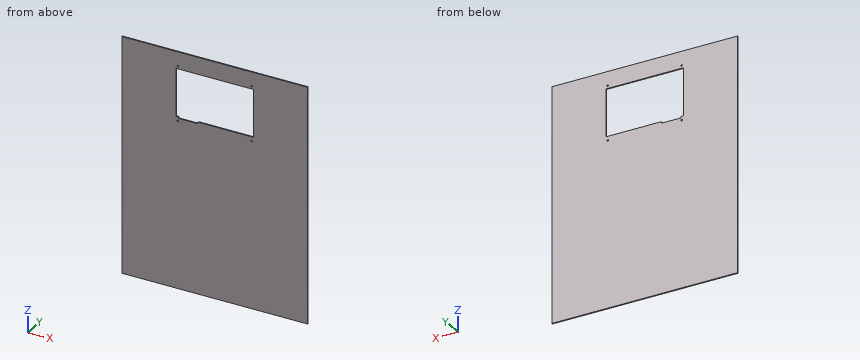
```python
from build123d import *

# Parameters (mm, degrees)
SKETCH1_W           = 395
SKETCH1_H           = 496
BOSS_EXTRUDE1_DEPTH = 2.5
CUT_EXTRUDE1_DEPTH  = 2.5
SKETCH6_R           = 1.65
CUT_EXTRUDE2_DEPTH  = 2.5


with BuildPart() as part:
    # Sketch1 → Boss-Extrude1 (new body)
    with BuildSketch(Plane(origin=(0, 0, 0), x_dir=(1, 0, 0), z_dir=(0, 1, 0))):
        Rectangle(SKETCH1_W, SKETCH1_H)
    extrude(amount=BOSS_EXTRUDE1_DEPTH)

    # Sketch4 → Cut-Extrude1 (cut)
    with BuildSketch(Plane(origin=(0, 2.5, 0), x_dir=(1, 0, 0), z_dir=(0, 1, 0))):
        with BuildLine():
            Line((-78.7, -112.1), (-82.2, -112.1))
            ThreePointArc((-82.2, -112.1), (-82.553553391, -112.246446609), (-82.7, -112.6))
            Line((-82.7, -112.6), (-82.7, -212))
            ThreePointArc((-82.7, -212), (-82.553553391, -212.353553391), (-82.2, -212.5))
            Line((-82.2, -212.5), (82.2, -212.5))
            ThreePointArc((82.2, -212.5), (82.553553391, -212.353553391), (82.7, -212))
            Line((82.7, -212), (82.7, -112.6))
            ThreePointArc((82.7, -112.6), (82.553553391, -112.246446609), (82.2, -112.1))
            Line((82.2, -112.1), (-34.7, -112.1))
            ThreePointArc((-34.7, -112.1), (-35.407106781, -111.807106781), (-35.7, -111.1))
            Line((-35.7, -111.1), (-35.7, -109.8))
            ThreePointArc((-35.7, -109.8), (-35.992893219, -109.092893219), (-36.7, -108.8))
            Line((-36.7, -108.8), (-76.7, -108.8))
            ThreePointArc((-76.7, -108.8), (-77.407106781, -109.092893219), (-77.7, -109.8))
            Line((-77.7, -109.8), (-77.7, -111.1))
            ThreePointArc((-77.7, -111.1), (-77.992893219, -111.807106781), (-78.7, -112.1))
        make_face()
    extrude(amount=-CUT_EXTRUDE1_DEPTH, mode=Mode.SUBTRACT)

    # Sketch6 → Cut-Extrude2 (cut)
    with BuildSketch(Plane(origin=(0, 2.5, 0), x_dir=(1, 0, 0), z_dir=(0, 1, 0))):
        with Locations((78.5, -103.4)):
            Circle(SKETCH6_R)
        with Locations((-78.5, -103.4)):
            Circle(SKETCH6_R)
        with Locations((-78.5, -218.3)):
            Circle(SKETCH6_R)
        with Locations((78.5, -218.3)):
            Circle(SKETCH6_R)
    extrude(amount=-CUT_EXTRUDE2_DEPTH, mode=Mode.SUBTRACT)


solid = part.part
```
Model file for the job. Use its own axes, mm. Coordinates: 2 decimals unless noted, no trailing zeros. Write each loop counter-clockwise with the first axis right and the second up, starting at its lowest first coordinate (ties: lowest second). Pieces come first, ordered by that corner, then holes. Notation, with made-up numbers: (51, -14) - (71, -14) arc R17 ccw to (71, -7) - close; hole circle Ø4 at (-2.5, -10.75). An arc over 180 degrees is marked (long way). One line per question, with ' | ' between items. Start each with the question number.
Q1. Cut at B-B, the plane x = -45.5. List the corners of the cut face in (y, z).
Q2. Pin check, flat tips, straight feed: pin 1 (2.5 mm diameter, centred on x = -78.5, z = 218.3, fed in from -Y); pin 2 (5.5 mm diameter, centred on x = 78.5, z = 218.3, fed in from +Y). Stop position of each tip, or through.
Q3. Drill centre lines: line 1 (Z direction, x = -78.5, y = 0.6); line 2 (X direction, y = 0.6, z = 103.4); line 3 (Z direction, x = 36, y = 1.6). Where is each one in solid material? Low to high. Write a range as [from, to].
Q4. Cut at A-A, the plane y = 1.05. List the corners of the cut face in (x, z).
Answer below:
1) outline: (0, -248) - (2.5, -248) - (2.5, 108.8) - (0, 108.8) - close; (0, 212.5) - (2.5, 212.5) - (2.5, 248) - (0, 248) - close
2) pin 1: through | pin 2: y = 2.5
3) line 1: [-248, 101.75], [105.05, 112.08], [212.5, 216.65], [219.95, 248] | line 2: [-197.5, -80.15], [-76.85, 76.85], [80.15, 197.5] | line 3: [-248, 112.1], [212.5, 248]
4) outline: (-197.5, -248) - (197.5, -248) - (197.5, 248) - (-197.5, 248) - close; hole (-82.7, 112.6) arc R0.5 ccw to (-82.2, 112.1) - (-78.7, 112.1) arc R1 cw to (-77.7, 111.1) - (-77.7, 109.8) arc R1 ccw to (-76.7, 108.8) - (-36.7, 108.8) arc R1 ccw to (-35.7, 109.8) - (-35.7, 111.1) arc R1 cw to (-34.7, 112.1) - (82.2, 112.1) arc R0.5 ccw to (82.7, 112.6) - (82.7, 212) arc R0.5 ccw to (82.2, 212.5) - (-82.2, 212.5) arc R0.5 ccw to (-82.7, 212) - close; hole circle Ø3.3 at (-78.5, 103.4); hole circle Ø3.3 at (-78.5, 218.3); hole circle Ø3.3 at (78.5, 103.4); hole circle Ø3.3 at (78.5, 218.3)
